Geometry: final body of the model. Coordinates: model frame, mm. A direction names the side the tool comes from. Coordinates: 2 decimals unless noted, no trailing zeros. Loops run counter-clockwise (first coordinate to the right, second up) from the corner with the lowest first, then second, coordinate; pieces in that order, holes last. Notation, with made-up numbers: (9.25, 59) -> (67.25, 59) arc R22 cw to (67.25, 87) -> close; hole circle Ø3 at (79, 11). An arc over 180 degrees is marked (long way). One line per item, written item: value. Start each with the question number.
from build123d import *

# Parameters (mm, degrees)
SKETCH1_R           = 1.5875
BOSS_EXTRUDE1_DEPTH = 5.08
FILLET1_R           = 2.54
FILLET2_R           = 0.762
SKETCH2_R           = 1.5875
CUT_EXTRUDE1_DEPTH  = 263.560055455


with BuildPart() as part:
    # Sketch1 → Boss-Extrude1 (new body)
    with BuildSketch(Plane(origin=(0, 0, 0), x_dir=(1, 0, 0), z_dir=(0, 1, 0))):
        Polygon((-29.21, -190.5), (-29.21, 190.5), (-38.1, 259.781963021), (38.1, 259.781963021), (29.21, 190.5), (29.21, -190.5), (38.1, -259.781963021), (-38.1, -259.781963021), align=None)
        with Locations(Location((-18.796, 102.235, 0), (0, 0, 270))):
            Circle(SKETCH1_R, mode=Mode.SUBTRACT)
        with Locations(Location((18.796, 102.235, 0), (0, 0, 90))):
            Circle(SKETCH1_R, mode=Mode.SUBTRACT)
        with Locations(Location((18.796, -102.235, 0), (0, 0, 270))):
            Circle(SKETCH1_R, mode=Mode.SUBTRACT)
        with Locations(Location((-18.796, -102.235, 0), (0, 0, 90))):
            Circle(SKETCH1_R, mode=Mode.SUBTRACT)
    extrude(amount=BOSS_EXTRUDE1_DEPTH)

    # Fillet1
    fillet1_edges = [part.edges().sort_by_distance(p)[0] for p in [
        (29.21, 2.54, -190.5),
        (29.21, 2.54, 190.5),
        (38.1, 2.54, 259.781963021),
        (-38.1, 2.54, 259.781963021),
        (-29.21, 2.54, 190.5),
        (-38.1, 2.54, -259.781963021),
        (38.1, 2.54, -259.781963021),
    ]]
    fillet(fillet1_edges, radius=FILLET1_R)

    # Fillet2
    fillet2_edges = [part.edges().sort_by_distance(p)[0] for p in [
        (-29.21, 0, -0.08114814),
        (-29.21, 5.08, -0.08114814),
        (-33.471297825, 0, -223.709345147),
        (-33.471297825, 5.08, -223.709345147),
        (33.48162577, 0, -223.78983337),
        (29.21, 0, 0),
        (33.48162577, 0, 223.78983337),
        (0, 0, 259.781963021),
        (-33.48162577, 0, 223.78983337),
        (0, 0, -259.781963021),
        (37.120174812, 0, -258.919831799),
        (37.120174812, 0, 258.919831799),
        (-37.120174812, 0, 258.919831799),
        (-37.120174812, 0, -258.919831799),
        (0, 5.08, -259.781963021),
        (33.48162577, 5.08, -223.78983337),
        (-33.48162577, 5.08, 223.78983337),
        (0, 5.08, 259.781963021),
        (33.48162577, 5.08, 223.78983337),
        (29.21, 5.08, 0),
        (37.120174812, 5.08, -258.919831799),
        (37.120174812, 5.08, 258.919831799),
        (-37.120174812, 5.08, 258.919831799),
        (-37.120174812, 5.08, -258.919831799),
        (-29.215169233, 0, 190.499669706),
        (-29.215169233, 5.08, 190.499669706),
        (29.215169233, 0, 190.499669706),
        (29.215169233, 5.08, 190.499669706),
        (29.215169233, 0, -190.499669706),
        (29.215169233, 5.08, -190.499669706),
    ]]
    fillet(fillet2_edges, radius=FILLET2_R)

    # Sketch2 → Cut-Extrude1 (cut, through all)
    with BuildSketch(Plane(origin=(0, 5.08, 0), x_dir=(1, 0, 0), z_dir=(0, 1, 0))):
        with Locations(Location((-12.7, 233.619963021, 0), (0, 0, 270))):
            Circle(SKETCH2_R)
        with Locations(Location((12.7, 233.619963021, 0), (0, 0, 90))):
            Circle(SKETCH2_R)
        with Locations(Location((11.833787679, -233.559959271, 0), (0, 0, 270))):
            Circle(SKETCH2_R)
        with Locations(Location((-13.566037681, -233.46576979, 0), (0, 0, 90))):
            Circle(SKETCH2_R)
    extrude(amount=-CUT_EXTRUDE1_DEPTH, mode=Mode.SUBTRACT)


solid = part.part
1. Section B-B on y = 2.95. Count the separate pieces of the cut face and the enclosed holes in it, plus the area to 3 significant figures.
2. Draft query along Z for faces 1 (the face through (33.422, 2.515, 223.326)), 2 (the face through (1, 5.08, -4)), 3 (the face through (-33.312, 0.229, -224.178)). Return one class per face: released by +Z, released by -Z, zero draft, split by the parting line, or undercut.
3. Set-up query: faces 4 (the face through (33.54, 2.52, -224.25)), 5 (the face through (-33.41, 2.52, -223.24)), 6 (the face through (33.326, 4.851, 224.281)), 7 (the face through (-33.207, 0.229, 223.354)). Return all of +Z, -Z, +X, -X, +Y, -Y with unobstructed straight access to the full face (end or side cutting, diameter ignored); none if empty.
4. Line query: L1, parallel to Z at x = 20, y = 4.7; L2, parallel to Z at x = 12.7, y = 1.3; L3, parallel to X at y = 4.7, z = 234.5. Output: solid intervals per line, ascending. Write a range as [from, to].
5. Pin query (flat end, axial travel): pin 1 Ø3.5 at (x, z) = (-18.796, 102.235) entering from +Y; pin 2 Ø2 at (y, z) = (4.5, 98) entering from -X. Return the tip coordinate at first contact, or that it passes through.
6. Section A-A on z = -118.5. Return the cut outline in (x, y), plus the area to 3 significant figures.
Checks:
1. separate pieces: 1
1. enclosed holes: 8
1. area: 31,500 mm²
2. face 1: undercut
2. face 2: zero draft
2. face 3: undercut
3. face 4: +X, +Y, -Y
3. face 5: -X, +Y, -Y
3. face 6: +X, +Y
3. face 7: -X, -Y
4. L1: [-259.68, -103.27], [-101.2, 101.2], [103.27, 259.68]
4. L2: [-259.78, -235.21], [-232.03, 232.23], [234.89, 259.78]
4. L3: [-34.75, -14.77], [-12.36, 10.55], [13.11, 34.75]
5. pin 1: y = 5.08
5. pin 2: x = -29.21
6. outline: (-29.21, 0.76) arc R0.76 ccw to (-28.45, 0) -> (28.45, 0) arc R0.76 ccw to (29.21, 0.76) -> (29.21, 4.32) arc R0.76 ccw to (28.45, 5.08) -> (-28.45, 5.08) arc R0.76 ccw to (-29.21, 4.32) -> close
6. area: 296 mm²
